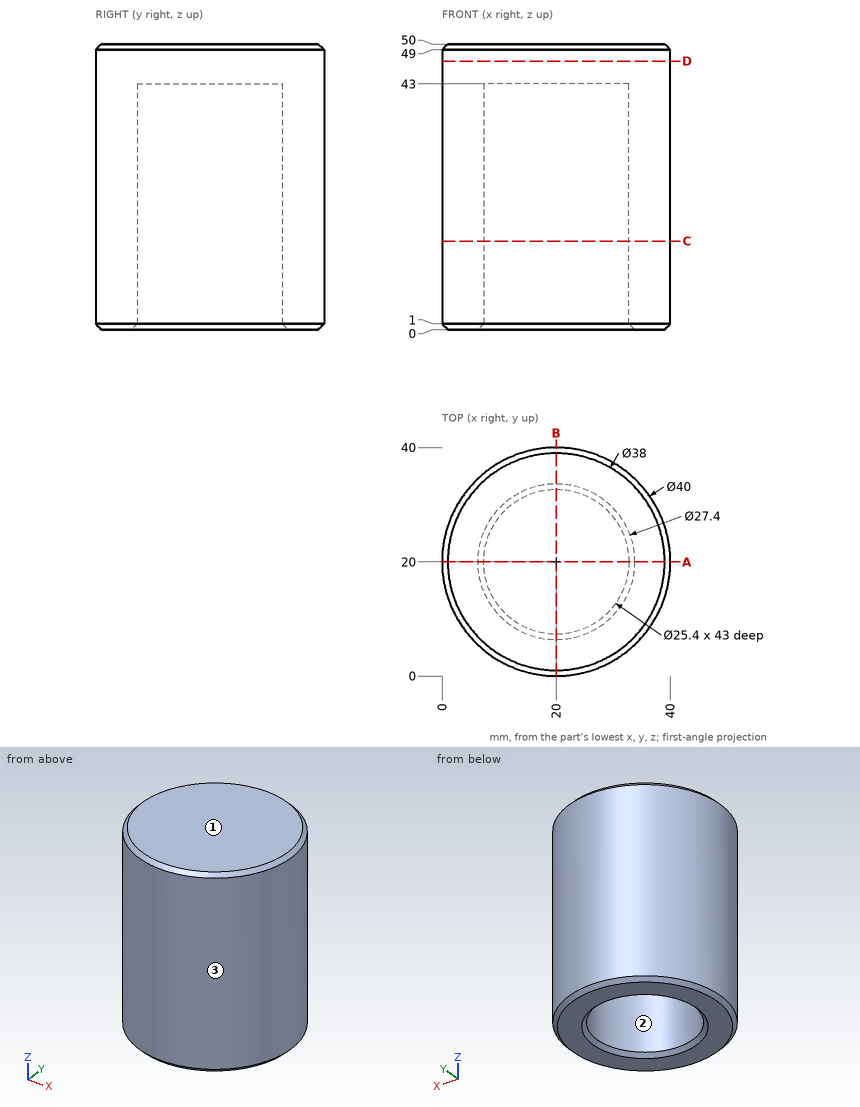
For this review, use the dimensioned drawing (mm, ordinates from the lowest corner) and the shaded views. Round coordinates to 2 decimals unless told otherwise and drop trailing zeros. Order: outer loops, then holes, each group sorted by start corner. A loop starts at its lowest first (then second) coordinate and runs counter-clockwise, first axis right, second up.
1) Consider section A-A (y = 20). State the section outline as (x, z) points, plus the area to 3 significant figures.
The answers:
outline: (0, 1) - (1, 0) - (6.3, 0) - (7.3, 1) - (7.3, 43) - (32.7, 43) - (32.7, 1) - (33.7, 0) - (39, 0) - (40, 1) - (40, 49) - (39, 50) - (1, 50) - (0, 49) - close
area: 905 mm2
2) For L1, parallel to Y at x = 20, z = 11.5; L2, parallel to Z at x = 22.5, y = 25.5; L3, parallel to Y at x = 29, z = 38.5, list the stretches that pass through material, from the lowest coordinate up.
The answers:
L1: y = 0 to 7.3, 32.7 to 40
L2: z = 43 to 50
L3: y = 2.14 to 11.04, 28.96 to 37.86
3) Consider section C-C (z = 15.5). State the section outline as (x, y) points, plus the area to 3 significant figures.
The answers:
outline: circle Ø40 at (20, 20); hole circle Ø25.4 at (20, 20)
area: 750 mm2
4) Clearance check with flat-ended pins moving along their axes: pin 1 Ø1 at (x, z) = (27.5, 34) entering from -Y (3 decimals); pin 2 Ø10 at (y, z) = (32.5, 9.5) entering from +X; pin 3 Ø5 at (x, y) = (35, 23) entering from -Z; pin 4 Ø3 at (y, z) = (10.5, 30.5) entering from -X. State where each tip first meets the part, or that it passes through.
The answers:
pin 1: stops at y = 1.265
pin 2: stops at x = 38.54
pin 3: stops at z = 0
pin 4: stops at x = 1.67
5) Consider section D-D (z = 47). State the section outline as (x, y) points.
The answers:
outline: circle Ø40 at (20, 20)
6) Draft analysis for pull direction X (two halves, no side actions). For the marked faces 1, 2 and 3, state which applies: released by +X, released by -X, zero draft, split by the parting line, or undercut.
The answers:
face 1: zero draft
face 2: undercut
face 3: split by the parting line
